```python
from build123d import *

# Parameters (mm, degrees)
SKETCH_1_W          = 18
SKETCH_1_H          = 35
EXTRUDE_1_DEPTH     = 10
SKETCH_2_W          = 17
SKETCH_2_H          = 5
CUT_EXTRUDE_2_DEPTH = 41.607881008
SKETCH_3_R          = 2.5
CUT_EXTRUDE_1_DEPTH = 41.607881008
CHAMFER_1_SIZE      = 3


with BuildPart() as part:
    # Эскиз1 → Вытянуть1 (new body)
    with BuildSketch(Plane(origin=(0, 0, 0), x_dir=(1, 0, 0), z_dir=(0, 1, 0))):
        with Locations((9, -17.5)):
            Rectangle(SKETCH_1_W, SKETCH_1_H)
    extrude(amount=EXTRUDE_1_DEPTH)

    # Эскиз2 → Вытянуть2 (cut, through all)
    with BuildSketch(Plane(origin=(18, 0, 0), x_dir=(0, 0, -1), z_dir=(1, 0, 0))):
        with Locations((-26.5, 2.5)):
            Rectangle(SKETCH_2_W, SKETCH_2_H)
    extrude(amount=-CUT_EXTRUDE_2_DEPTH, mode=Mode.SUBTRACT)

    # Эскиз3 → Вырез-Вытянуть1 (cut, through all)
    with BuildSketch(Plane.ZY):
        with Locations((4.695559751, 5)):
            Circle(SKETCH_3_R)
    extrude(amount=-CUT_EXTRUDE_1_DEPTH, mode=Mode.SUBTRACT)

    # Фаска1
    chamfer_1_edges = [part.edges().sort_by_distance(p)[0] for p in [
        (9, 10, 0),
        (9, 0, 0),
    ]]
    chamfer(chamfer_1_edges, length=CHAMFER_1_SIZE)


solid = part.part
```
Check sheet for the modelled part. Datum: model origin and axes. Units: mm. A direction names the side the tool comes from. Round coordinates to 2 decimals unless told otherwise and drop trailing zeros. Write each loop counter-clockwise with the first axis right and the second up, starting at its lowest first coordinate (ties: lowest second). Pieces come first, ordered by that corner, then holes. Notation, with made-up numbers: (54, -14) -> (87, -14) arc R24 ccw to (87, 18) -> close; hole circle Ø2 at (88.5, 57). An arc over 180 degrees is marked (long way). One line per question, with ' | ' between items. Start each with the question number.
1. Set-up check for faces 5 (the face through (9, 5, 27)), 6 (the face through (9, 0, 10)): record each of +Z, -Z, +X, -X, +Y, -Y from which the full face is reachable in a straight line by a thin tool's end or side.
2. Sectioned sample at B-B, the plane y = 5.5. Record the cut outline in (x, z).
3. Release check for a two-part mould opening along Y. For faces 1 (the face through (9, 7, 35)), 2 (the face through (9, 10, 19)), 3 (the face through (9, 2, 1)), 4 (the face through (8.87, 7.48, 4.37)) record: +Y half, -Y half, draft (parallel to the pull), parting line (faces both ways), or undercut.
4. Sectioned sample at A-A, the plane x = 9. Record the cut outline in (y, z).
5. Scan lines: line 1 along Y through (x, z) = (14, 5.5); line 2 along Z through (x, y) = (16.75, 3.75); line 3 along Y through (x, z) = (5.5, 32). Record each from-to range of solid material in increasing order. Write a range as from..to.
6. Sectioned sample at C-C, the plane y = 2. Record the cut outline in (x, z), then the cut area to 3 significant figures.
7. Depth check by flat-ended pin: pin 1 (2.5 mm diameter, centred on x = 4.5, y = 2, fed in from +Z); pin 2 (6 mm diameter, centred on y = 5.5, z = 13, fed in from -X); pin 3 (1 mm diameter, centred on x = 7.5, z = 21.5, fed in from -Y); pin 4 (4.5 mm diameter, centred on y = 5, z = 4.7, fed in from +X) (3 decimals). Enter the tip coordinate at first touch or a pass-through.
Taken from the geometry:
1) face 5: +Z, +X, -X, -Y | face 6: +Z, -Z, +X, -X, -Y
2) outline: (0, 0) -> (18, 0) -> (18, 2.25) -> (0, 2.25) -> close; (0, 7.15) -> (18, 7.15) -> (18, 35) -> (0, 35) -> close
3) face 1: draft | face 2: +Y half | face 3: -Y half | face 4: undercut
4) outline: (0, 3) -> (3, 0) -> (7, 0) -> (10, 3) -> (10, 35) -> (5, 35) -> (5, 18) -> (0, 18) -> close; hole circle Ø5 at (5, 4.7)
5) line 1: y = 0..2.63, 7.37..10 | line 2: z = 0..2.53, 6.86..18 | line 3: y = 5..10
6) outline: (0, 1) -> (18, 1) -> (18, 18) -> (0, 18) -> close | area: 306 mm^2
7) pin 1: stops at z = 18 | pin 2: stops at x = 0 | pin 3: stops at y = 5 | pin 4: passes through
